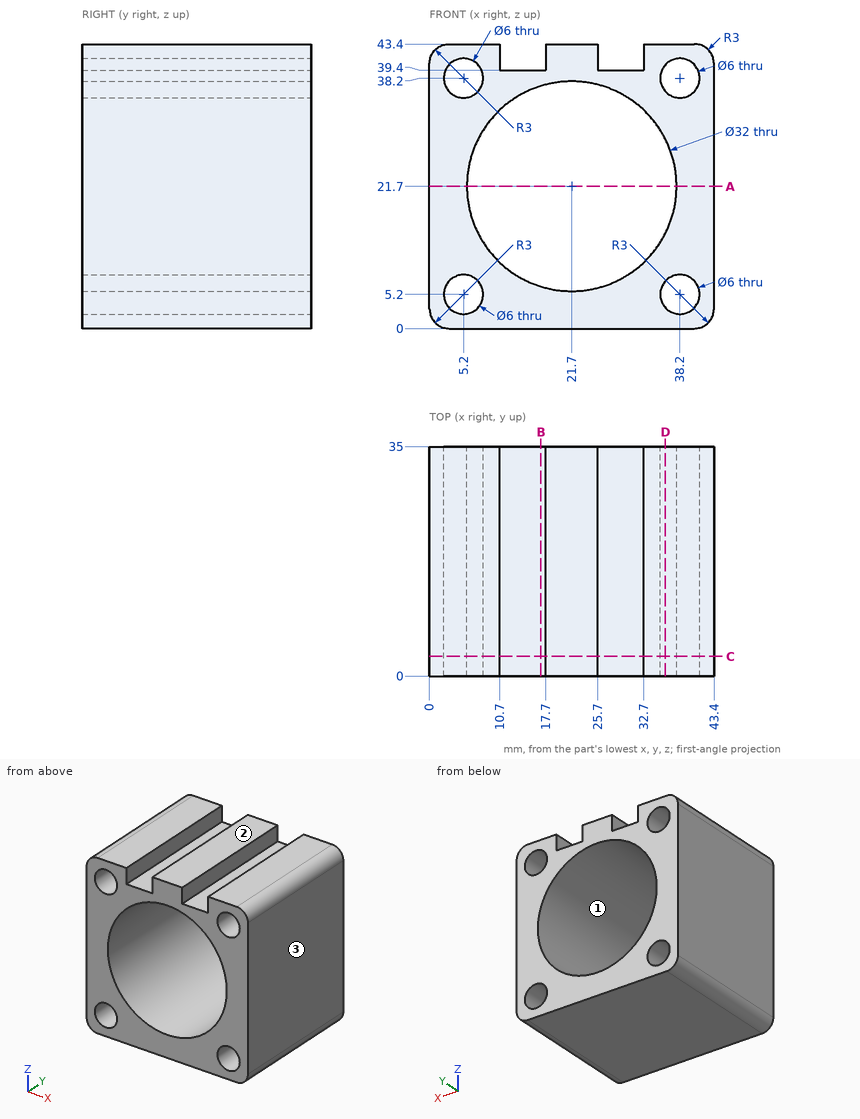
Input: dimensioned drawing with shaded views. Units: mm. Origin: part minimum x, y, z. Round coordinates to 2 decimals unless told otherwise and drop trailing zeros. Order: outer loops, then holes, each group sorted by start corner. A loop starts at its lowest first (then second) coordinate and runs counter-clockwise, first axis right, second up.
1. Material intervals for line 1 (Z direction, x = 5, y = 24); line 2 (X direction, y = 31, z = 21.5); line 3 (Z direction, x = 7.5, y = 27), sorted ascending.
The answers:
line 1: z = 0 to 2.21, 8.19 to 35.21, 41.19 to 43.4
line 2: x = 0 to 5.7, 37.7 to 43.4
line 3: z = 0 to 3.27, 7.13 to 14.33, 29.07 to 36.27, 40.13 to 43.4
2. Pin query (flat end, axial travel): P1, Ø2, axis at x = 29.5, y = 21, coming from the +Z side. Return the tip coordinate at first contact, or that it passes through.
The answers:
P1: stops at z = 39.4
3. Cut plane A-A, the plane z = 21.7. Output: boundary loops of the cut face in (x, y), then the cut area to 3 significant figures.
The answers:
outline: (0, 0) - (5.7, 0) - (5.7, 35) - (0, 35) - close; (37.7, 0) - (43.4, 0) - (43.4, 35) - (37.7, 35) - close
area: 399 mm2
4. Cut plane D-D, the plane x = 36. Output: boundary loops of the cut face in (y, z), then the cut area to 3 significant figures.
The answers:
outline: (0, 0) - (35, 0) - (35, 3.16) - (0, 3.16) - close; (0, 7.24) - (35, 7.24) - (35, 14.52) - (0, 14.52) - close; (0, 28.88) - (35, 28.88) - (35, 36.16) - (0, 36.16) - close; (0, 40.24) - (35, 40.24) - (35, 43.4) - (0, 43.4) - close
area: 731 mm2
5. Cut plane B-B, the plane x = 17. Output: boundary loops of the cut face in (y, z).
The answers:
outline: (0, 0) - (35, 0) - (35, 6.41) - (0, 6.41) - close; (0, 36.99) - (35, 36.99) - (35, 39.4) - (0, 39.4) - close
6. Mould query, pull axis Z, two halves, no side actions, for the marked faces 1, 2 and 3. Classes: released by +Z, released by -Z, zero draft, split by the parting line, or undercut.
The answers:
face 1: undercut
face 2: released by +Z
face 3: zero draft
7. Cut plane C-C, the plane y = 3. Output: boundary loops of the cut face in (x, z), then the cut area to 3 significant figures.
The answers:
outline: (0, 3) arc R3 ccw to (3, 0) - (40.4, 0) arc R3 ccw to (43.4, 3) - (43.4, 40.4) arc R3 ccw to (40.4, 43.4) - (32.7, 43.4) - (32.7, 39.4) - (25.7, 39.4) - (25.7, 43.4) - (17.7, 43.4) - (17.7, 39.4) - (10.7, 39.4) - (10.7, 43.4) - (3, 43.4) arc R3 ccw to (0, 40.4) - close; hole circle Ø6 at (5.2, 5.2); hole circle Ø6 at (5.2, 38.2); hole circle Ø32 at (21.7, 21.7); hole circle Ø6 at (38.2, 5.2); hole circle Ø6 at (38.2, 38.2)
area: 902 mm2
